Verification items for the finished model (mm, model axes). Face numbers are marked on the shaded views. A direction names the side the tool comes from. Round coordinates to 2 decimals unless told otherwise and drop trailing zeros. Order: outer loops, then holes, each group sorted by start corner. A loop starts at its lowest first (then second) coordinate and runs counter-clockwise, first axis right, second up. Notation, with made-up numbers: (23.25, 33) -> (57.25, 33) arc R27 cw to (57.25, 65) -> close; hole circle Ø10 at (60, 43.5). An arc over 180 degrees is marked (long way). Answer in a Markdown table with one row per item. Add a question column.
```python
from build123d import *

# Parameters (mm, degrees)
F1_DEPTH = 25.4
F0_R     = 19.05
F2_DEPTH = 38.1
F0_R_2   = 6.35
F3_DEPTH = 31.75


with BuildPart() as f1:
    # F0 (on Top) → F1 (new body)
    with BuildSketch(Plane.XY):
        with BuildLine():
            ThreePointArc((-55.567108, 34.004813), (-39.269963, 25.77097), (-32.707108, 8.732132))
            ThreePointArc((-32.707108, 8.732132), (-39.269963, -8.306706), (-55.567108, -16.540549))
            Line((-55.567108, -16.540549), (70.162892, -3.904209))
            ThreePointArc((70.162892, -3.904209), (56.192892, 8.732132), (70.162892, 21.368472))
            Line((70.162892, 21.368472), (-55.567108, 34.004813))
        make_face()
        with BuildLine():
            ThreePointArc((-20.007108, 2.382132), (-26.357108, 8.732132), (-20.007108, 15.082132))
            Line((-20.007108, 15.082132), (30.792892, 15.082132))
            ThreePointArc((30.792892, 15.082132), (35.28302, 13.22226), (37.142892, 8.732132))
            ThreePointArc((37.142892, 8.732132), (35.28302, 4.242004), (30.792892, 2.382132))
            Line((30.792892, 2.382132), (-20.007108, 2.382132))
        make_face(mode=Mode.SUBTRACT)
    extrude(amount=F1_DEPTH)

    # F0 (on Top) → F2 (join)
    with BuildSketch(Plane.XY):
        with BuildLine():
            ThreePointArc((-55.567108, -16.540549), (-39.269963, -8.306706), (-32.707108, 8.732132))
            ThreePointArc((-32.707108, 8.732132), (-39.269963, 25.77097), (-55.567108, 34.004813))
            ThreePointArc((-55.567108, 34.004813), (-83.507108, 8.732132), (-55.567108, -16.540549))
        make_face()
        with Locations((-58.107108, 8.732132)):
            Circle(F0_R, mode=Mode.SUBTRACT)
    extrude(amount=F2_DEPTH)

    # F0 (on Top) → F3 (join)
    with BuildSketch(Plane.XY):
        with BuildLine():
            ThreePointArc((81.592892, 8.732132), (78.311464, 17.251551), (70.162892, 21.368472))
            ThreePointArc((70.162892, 21.368472), (56.192892, 8.732132), (70.162892, -3.904209))
            ThreePointArc((70.162892, -3.904209), (78.311464, 0.212713), (81.592892, 8.732132))
        make_face()
        with Locations((68.892892, 8.732132)):
            Circle(F0_R_2, mode=Mode.SUBTRACT)
    extrude(amount=F3_DEPTH)


solid = f1.part
```
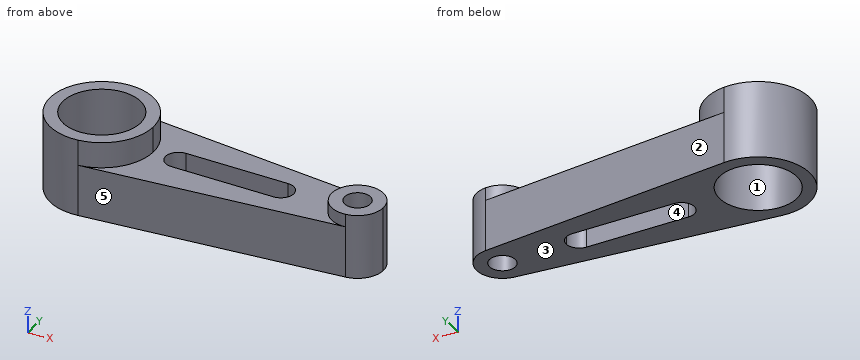
1) Draft check along X on the marked faces 1, 2 and 3. Enter one of: +X half, -X half, draft (parallel to the pull), parting line (faces both ways), or undercut.
2) Tool access check on the marked faces 4 and 5. Record the directions out of +Z, -Z, +X, -X, +Y, -Y that give a thin tool (end or side, any length) a straight path to the whole face; none if there is none.
3) Cross-section at B-B, the plane y = 4.5. Record the boundary of the cut face in (x, z), and give its area (3 significant figures).
4) Cross-section at C-C, the plane z = 18.5. Record the boundary of the cut face in (x, y).
5) Cross-section at A-A, the plane z = 29.5. Record the boundary of the cut face in (x, y).
6) Depth check by flat-ended pin: P1, Ø12.5, axis at x = 0, z = 17.5, coming from the -Y side; P2, Ø1, axis at y = -2, z = 19, coming from the +X side; P3, Ø7.5, axis at x = -1.5, z = 17.5, coming from the +Y side; P4, Ø7.5, axis at x = 68.89, y = 8.73, coming from the +Z side. Enter the tip coordinate at first touch or a pass-through.
7) Thickness scan on L1, parallel to X at y = 18, z = 31.5; L2, parallel to X at y = 13, z = 29; L3, parallel to X at y = 11, z = 7. Record the ranges inside material, lowest first. Write a range as [from, to].
8) Cross-section at D-D, the plane x = 8. Record the boundary of the cut face in (y, z).
Results below:
| question | item | result |
|---|---|---|
| 1 | face 1 | undercut |
| 1 | face 2 | +X half |
| 1 | face 3 | draft |
| 2 | face 4 | +Z, -Z |
| 2 | face 5 | +Z, -Z, +X, -Y |
| 3 | outline | (-83.15, 0) -> (-76.68, 0) -> (-76.68, 38.1) -> (-83.15, 38.1) -> close; (-39.53, 0) -> (-24.74, 0) -> (-24.74, 25.4) -> (-33.06, 25.4) -> (-33.06, 38.1) -> (-39.53, 38.1) -> close; (35.53, 0) -> (64.16, 0) -> (64.16, 31.75) -> (56.92, 31.75) -> (56.92, 25.4) -> (35.53, 25.4) -> close; (73.63, 0) -> (80.87, 0) -> (80.87, 31.75) -> (73.63, 31.75) -> close |
| 3 | area | 1,710 mm² |
| 4 | outline | (-55.57, -16.54) -> (70.16, -3.9) arc R12.7 ccw to (81.59, 8.73) arc R12.7 ccw to (70.16, 21.37) -> (-55.57, 34) arc R25.4 ccw (long way) to start; hole circle Ø38.1 at (-58.11, 8.73); hole (-20.01, 2.38) -> (30.79, 2.38) arc R6.35 ccw to (30.79, 15.08) -> (-20.01, 15.08) arc R6.35 ccw to start; hole circle Ø12.7 at (68.89, 8.73) |
| 5 | outline | (-55.57, -16.54) arc R25.4 ccw to (-32.71, 8.73) arc R25.4 ccw to (-55.57, 34) arc R25.4 ccw (long way) to start; (70.16, -3.9) arc R12.7 ccw to (81.59, 8.73) arc R12.7 ccw (long way) to start; hole circle Ø38.1 at (-58.11, 8.73); hole circle Ø12.7 at (68.89, 8.73) |
| 6 | P1 | y = -11.58 |
| 6 | P2 | x = 76.42 |
| 6 | P3 | y = 28.95 |
| 6 | P4 | through |
| 7 | L1 | [-81.76, -74.75], [-41.46, -34.46], [60.21, 77.58] |
| 7 | L2 | [-83.15, -76.67], [-39.54, -33.07], [56.93, 64.19], [73.59, 80.85] |
| 7 | L3 | [-83.41, -77.02], [-39.19, -25.94], [36.72, 62.96], [74.82, 81.39] |
| 8 | outline | (-10.15, 0) -> (2.38, 0) -> (2.38, 25.4) -> (-10.15, 25.4) -> close; (15.08, 0) -> (27.62, 0) -> (27.62, 25.4) -> (15.08, 25.4) -> close |
